Autodesk Inventor part; units mm, degrees
ref_plane "YZ Plane" through (0, 0, 0) normal (1, 0, 0) x (0, 1, 0)
ref_plane "XZ Plane" through (0, 0, 0) normal (0, 1, 0) x (-1, 0, 0)
ref_plane "XY Plane" through (0, 0, 0) normal (0, 0, 1) x (1, 0, 0)
sketch "Sketch1" plane through (0, 0, 0) normal (0, 0, 1) x (1, 0, 0)
  line L0 (0, 0) -> (330, 0)
  line L1 (330, 0) -> (330, 510)
  line L2 (330, 510) -> (0, 510)
  line L3 (0, 510) -> (0, 0)
  dimension "d0" = 330
  dimension "d1" = 510
extrude "Extrusion1" add sketch "Sketch1" along normal blind 150
sketch "Sketch2" plane through (0, 0, 0) normal (0, -1, 0) x (1, 0, 0)
  circle A0 centre (165, -304.672) radius 315
  line L0 (85, 0) -> (245, 0)
  line L1 (0, 0) -> (330, 0)
  circle A1 centre (165, -304.672) radius 317
  point P0 (165, 0)
  point P1 (165, 0)
  dimension "d4" = 630
  dimension "d8" = 160
  dimension "d9" = 2
extrude "Extrusion2" cut sketch "Sketch2" against normal through all
sketch "Sketch3" plane through (0, 0, 150) normal (0, 0, 1) x (1, 0, 0)
  line L0 (0, 0) -> (330, 0)
  line L1 (330, 0) -> (330, 510)
  line L2 (330, 510) -> (0, 510)
  line L3 (0, 510) -> (0, 0)
  line L4 (10, 10) -> (320, 10)
  line L5 (320, 10) -> (320, 500)
  line L6 (320, 500) -> (10, 500)
  line L7 (10, 500) -> (10, 10)
  dimension "d10" = 10
extrude "Extrusion3" cut sketch "Sketch3" against normal blind 130 contours L7 L6 L5 L4
sketch "Sketch4" plane through (0, 0, 20) normal (0, 0, 1) x (1, 0, 0)
  line L0 (10, 500) -> (320, 500) construction
  line L1 (85, 500) -> (245, 500) construction
  line L2 (245, 500) -> (245, 10) construction
  line L3 (245, 10) -> (85, 10) construction
  line L4 (85, 10) -> (85, 500) construction
  line L5 (320, 10) -> (10, 10) construction
  line L6 (85, 500) -> (245, 500) construction
  line L7 (245, 500) -> (245, 455) construction
  line L8 (245, 455) -> (85, 455) construction
  line L9 (85, 455) -> (85, 500) construction
  line L10 (85, 455) -> (245, 455) construction
  line L11 (245, 455) -> (245, 400) construction
  line L12 (245, 400) -> (85, 400) construction
  line L13 (85, 400) -> (85, 455) construction
  line L14 (85, 400) -> (245, 400) construction
  line L15 (245, 400) -> (245, 345) construction
  line L16 (245, 345) -> (85, 345) construction
  line L17 (85, 345) -> (85, 400) construction
  line L18 (85, 345) -> (245, 345) construction
  line L19 (245, 345) -> (245, 290) construction
  line L20 (245, 290) -> (85, 290) construction
  line L21 (85, 290) -> (85, 345) construction
  line L22 (85, 290) -> (245, 290) construction
  line L23 (245, 290) -> (245, 235) construction
  line L24 (245, 235) -> (85, 235) construction
  line L25 (85, 235) -> (85, 290) construction
  circle A0 centre (130.3559, 262.5) radius 15
  circle A1 centre (199.6441, 262.5) radius 15
  line L26 (130.3559, 262.5) -> (199.6441, 262.5) construction
  point P0 (0, 0)
  point P1 (165, 500)
  point P2 (165, 500)
  point P3 (165, 262.5)
  point P4 (165, 235)
  point P5 (245, 262.5)
  dimension "d13" = 160
  dimension "d14" = 45
  dimension "d15" = 55
  dimension "d16" = 55
  dimension "d17" = 55
  dimension "d18" = 55
  dimension "d19" = 30
  dimension "d20" = 30
  dimension "d21" = 69.2883
extrude "Extrusion4" cut sketch "Sketch4" against normal through all
sketch "Sketch5" plane through (0, 0, 150) normal (0, 0, 1) x (1, 0, 0)
  line L0 (330, 510) -> (0, 510)
  line L1 (0, 0) -> (330, 0)
  line L2 (330, 510) -> (165, 510)
  line L3 (165, 510) -> (165, 0)
  line L4 (165, 0) -> (330, 0)
  line L5 (330, 0) -> (330, 510)
  line L6 (0, 510) -> (0, 0)
  line L7 (330, 0) -> (0, 0)
  line L8 (0, 0) -> (0, 340)
  line L9 (0, 340) -> (330, 340)
  line L10 (330, 340) -> (330, 0)
  dimension "d24" = 340
extrude "Extrusion5" cut sketch "Sketch5" against normal through all contours L5 L9 L3 L0 | L5 L1 L3 L9 | L3 L1 L6 L9
sketch "Sketch7" plane through (0, 510, 0) normal (-1, 0, 0) x (0, 0, 1)
  line L0 (20, -10) -> (31, -10)
  line L1 (31, -10) -> (31, -120)
  line L2 (31, -120) -> (20, -120)
  line L3 (20, -120) -> (20, -10)
  line L4 (0, 0) -> (150, 0)
  line L5 (0, 0) -> (0, -170)
  line L6 (20, -170) -> (20, -10)
  line L7 (20, -170) -> (20, -10)
  point P0 (0, -510)
  dimension "d31" = 10
  dimension "d32" = 20
  dimension "d33" = 11
  dimension "d34" = 110
extrude "Extrusion7" cut sketch "Sketch7" against normal through all
sketch "Sketch8" plane through (0, 510, 0) normal (-1, 0, 0) x (0, 0, 1)
  line L0 (150, -10) -> (31, -10)
  line L1 (36, -10) -> (64, -10)
  line L2 (64, -10) -> (64, -35)
  line L3 (64, -35) -> (36, -35)
  line L4 (36, -35) -> (36, -10)
  line L5 (31, -120) -> (31, -10)
  point P0 (0, -510)
  dimension "d37" = 28
  dimension "d38" = 25
  dimension "d39" = 5
extrude "Extrusion8" cut sketch "Sketch8" against normal through all
sketch "Sketch9" plane through (0, 510, 0) normal (-1, 0, 0) x (0, 0, 1)
  line L0 (36, -40) -> (51, -40)
  line L1 (51, -40) -> (51, -65)
  line L2 (51, -65) -> (36, -65)
  line L3 (36, -65) -> (36, -40)
  line L4 (36, -35) -> (64, -35)
  point P0 (0, -510)
  dimension "d42" = 15
  dimension "d43" = 25
  dimension "d44" = 5
extrude "Extrusion9" cut sketch "Sketch9" against normal through all
sketch "Sketch10" plane through (0, 510, 150) normal (0, 1, 0) x (1, 0, 0)
  circle A0 centre (120, 45) radius 22.5
  line L0 (165, 0) -> (165, 137.672)
  line L1 (10, 0) -> (165, 0)
  point P0 (0, 150)
  dimension "d47" = 45
  dimension "d48" = 45
  dimension "d49" = 45
extrude "Extrusion10" cut sketch "Sketch10" against normal through all
properties part number "CA002" material "ABS Plastic"
Verification items for the finished model (mm, model axes). A direction names the side the tool comes from. Give positions to 0.01 mm unless a question says otherwise; leave off trailing zeros. Order: outer loops, then holes, each group sorted by start corner. A loop starts at its lowest first (then second) coordinate and runs counter-clockwise, first axis right, second up. Notation, with made-up numbers: M -5.75,42.25 L 29.25,42.25 A24 cw 29.25,78.25 Z; hole C -10,48.25 d11. An arc over 180 degrees is marked long. Answer in a Markdown table with one row per item. Add a question column.
Item 1: Gauge pin test, flat ends, axial feed: pin 1 (1.5 mm diameter, centred on y = 388, z = 26, fed in from +X); pin 2 (4 mm diameter, centred on x = 57, y = 371.5, fed in from +Z); pin 3 (4 mm diameter, centred on x = 65.5, z = 40.5, fed in from -Y). Record the tip position at first contact, or that the pin passes through.
Item 2: Tool access check on faces 4 (the flat face through (45.4, 340, 19.8)), 5 (the flat face through (5, 390, 26)). Record the directions out of +Z, -Z, +X, -X, +Y, -Y that give a thin tool (end or side, any length) a straight path to the whole face; none if there is none.
Item 3: Section check A-A, the plane y = 420.5. Enter the section's corners in (x, z), and give its area (3 significant figures).
Item 4: Mould release check, pull along Z, two halves, no side actions. Record for faces 1 (the flat face through (5, 457, 36)), 2 (the flat face through (10, 421, 86)), 3 (the flat face through (38, 426, 0)): released by +Z, released by -Z, zero draft, split by the parting line, or undercut.
Item 5: Section check B-B, the plane z = 91.5. Enter the section's corners in (x, y), and give its area (3 significant figures).
Item 6: Section check C-C, the plane x = 120. Enter the section's corners in (y, z), and give its area (3 significant figures).
Item 7: Scan lines: probe 1 along X at (y, z) = (503.25, 105); probe 2 along Z at (x, y) = (52.5, 361.5); probe 3 along Z at (x, y) = (120, 507). Record each from-to range of solid material in increasing order. Write a range as from..to.
Item 8: Section check D-D, the plane z = 73. Enter the section's corners in (x, y), and give its area (3 significant figures).
Filled sheet:
| question | item | result |
|---|---|---|
| 1 | pin 1 | stops at x = 10 |
| 1 | pin 2 | stops at z = 20 |
| 1 | pin 3 | stops at y = 500 |
| 2 | face 4 | +Z, -Z, +X, -X, -Y |
| 2 | face 5 | +X, -X |
| 3 | outline | M 0,0 L 77.46,0 A317 cw 165,12.33 L 165,20 L 0,20 Z; M 0,31 L 10,31 L 10,150 L 0,150 Z |
| 3 | area | 3,770 mm^2 |
| 4 | face 1 | undercut |
| 4 | face 2 | zero draft |
| 4 | face 3 | released by -Z |
| 5 | outline | M 0,340 L 10,340 L 10,500 L 102,500 L 102,510 L 0,510 Z; M 138,500 L 165,500 L 165,510 L 138,510 Z |
| 5 | area | 2,890 mm^2 |
| 6 | outline | M 340,9.12 L 510,9.12 L 510,82.5 L 500,82.5 L 500,20 L 340,20 Z; M 500,127.5 L 510,127.5 L 510,150 L 500,150 Z |
| 6 | area | 2,700 mm^2 |
| 7 | probe 1 | x = 0..97.5, 142.5..165 |
| 7 | probe 2 | z = 0..20 |
| 7 | probe 3 | z = 9.12..82.5, 127.5..150 |
| 8 | outline | M 0,340 L 10,340 L 10,500 L 165,500 L 165,510 L 0,510 Z |
| 8 | area | 3,250 mm^2 |
